Model file for the job. Use its own axes, mm. Round coordinates to 2 decimals unless told otherwise and drop trailing zeros. Loops run counter-clockwise (first coordinate to the right, second up) from the corner with the lowest first, then second, coordinate; pieces in that order, holes last. Notation, with made-up numbers: (3.25, -35.5) - (37.25, -35.5) arc R10 ccw to (37.25, -27.5) - close; hole circle Ø3 at (63, -38). An arc over 180 degrees is marked (long way). Answer as a JSON object with one key per item and string values.
from build123d import *

# Parameters (mm, degrees)
SKETCH1_W           = 396.875
SKETCH1_H           = 298.45
BOSS_EXTRUDE1_DEPTH = 2.38125
SKETCH5_R           = 1
CUT_EXTRUDE4_DEPTH  = 10
SKETCH6_R           = 2
SKETCH6_R_2         = 30
CUT_EXTRUDE5_DEPTH  = 10
SKETCH7_R           = 12.7
CUT_EXTRUDE6_DEPTH  = 10
CUT_EXTRUDE7_DEPTH  = 10


with BuildPart() as part:
    # Sketch1 → Boss-Extrude1 (new body)
    with BuildSketch(Plane(origin=(0, 0, 0), x_dir=(1, 0, 0), z_dir=(0, 1, 0))):
        Rectangle(SKETCH1_W, SKETCH1_H)
    extrude(amount=BOSS_EXTRUDE1_DEPTH)

    # Sketch5 → Cut-Extrude4 (cut)
    with BuildSketch(Plane.XZ):
        with Locations(Location((-138.4375, 138.55, 0), (0, 0, 270))):
            Circle(SKETCH5_R)
        with Locations(Location((-138.4375, -138.55, 0), (0, 0, 270))):
            Circle(SKETCH5_R)
        with Locations(Location((-131.4375, -121.05, 0), (0, 0, 270))):
            Circle(SKETCH5_R)
        with Locations(Location((-131.4375, 121.05, 0), (0, 0, 270))):
            Circle(SKETCH5_R)
        with Locations(Location((-145.4375, 121.05, 0), (0, 0, 270))):
            Circle(SKETCH5_R)
        with Locations(Location((-145.4375, -121.05, 0), (0, 0, 270))):
            Circle(SKETCH5_R)
    extrude(amount=-CUT_EXTRUDE4_DEPTH, mode=Mode.SUBTRACT)

    # Sketch6 → Cut-Extrude5 (cut)
    with BuildSketch(Plane(origin=(0, 2.38125, 0), x_dir=(1, 0, 0), z_dir=(0, 1, 0))):
        with Locations(Location((123.4375, 52.475, 0), (0, 0, 270))):
            Circle(SKETCH6_R)
        with Locations(Location((123.4375, -37.525, 0), (0, 0, 270))):
            Circle(SKETCH6_R)
        with Locations(Location((168.4375, 7.475, 0), (0, 0, 270))):
            Circle(SKETCH6_R)
        with Locations(Location((78.4375, 7.475, 0), (0, 0, 270))):
            Circle(SKETCH6_R)
        with Locations(Location((123.4375, 7.475, 0), (0, 0, 270))):
            Circle(SKETCH6_R_2)
    extrude(amount=-CUT_EXTRUDE5_DEPTH, mode=Mode.SUBTRACT)

    # Sketch7 → Cut-Extrude6 (cut)
    with BuildSketch(Plane(origin=(0, 2.38125, 0), x_dir=(1, 0, 0), z_dir=(0, 1, 0))):
        with Locations(Location((153.4375, 84.225, 0), (0, 0, 270))):
            Circle(SKETCH7_R)
    extrude(amount=-CUT_EXTRUDE6_DEPTH, mode=Mode.SUBTRACT)

    # Sketch8 → Cut-Extrude7 (cut)
    with BuildSketch(Plane(origin=(0, 2.38125, 0), x_dir=(1, 0, 0), z_dir=(0, 1, 0))):
        Polygon((131.7625, -149.225), (198.4375, -82.55), (198.4375, -149.225), align=None)
        Polygon((198.4375, 149.225), (131.7625, 149.225), (198.4375, 82.55), align=None)
    cut_extrude7 = extrude(amount=-CUT_EXTRUDE7_DEPTH, mode=Mode.SUBTRACT)

    # Mirror1: Cut-Extrude7 across plane
    add(cut_extrude7.mirror(Plane(origin=(0, 0, 0), x_dir=(0, 0, 1), z_dir=(1, 0, 0))), mode=Mode.SUBTRACT)


solid = part.part
1) Two-plate mould, pull along Z, no slides. Class faces 1 (the flat face through (-3, 2.381, -2)), 2 (the flat face through (164.633, 1.207, 116.354)), 3 (the cylindrical face through (94.15, 1.21, -13.98)): pulls with the +Z half, pulls with the -Z half, needs draft (parallel to the pull), parting line crosses it, or undercut.
Values follow:
{"face 1": "needs draft", "face 2": "pulls with the +Z half", "face 3": "undercut"}
2) Slice it at A-A on y = 1.85. Count the separate pieces of the cut face and the enclosed holes in it, then the cut area to 3 significant figures.
Values follow:
{"separate pieces": "1", "enclosed holes": "12", "area": "106,000 mm²"}
3) Drop flat-ended pins along their axis: P1, Ø1.6, axis at x = -138.44, z = -138.55, coming from the +Y side; P2, Ø6.5, axis at x = 78.44, z = -7.48, coming from the -Y side. Give the stop position or say it passes through.
Values follow:
{"P1": "through", "P2": "y = 0"}
4) Slice it at C-C on x = -157.5. List the corners of the cut face in (y, z).
Values follow:
{"outline": "(0, -123.49) - (2.38, -123.49) - (2.38, 123.49) - (0, 123.49) - close"}
5) Probe probe 1 along X at (y, z) = (1.1, 121.05); probe 2 along Z at (x, y) = (-141.5, 1); probe 3 along X at (y, z) = (1.8, -4.5). List the from-to ranges inside material, lowest first.
Values follow:
{"probe 1": "-159.94 to -146.44, -144.44 to -132.44, -130.44 to 159.94", "probe 2": "-139.49 to 139.49", "probe 3": "-198.44 to 93.59, 153.29 to 198.44"}
6) Slice it at B-B on z = -127. List the corners of the cut face in (x, y), then the cut area to 3 significant figures.
Values follow:
{"outline": "(-153.99, 0) - (153.99, 0) - (153.99, 2.38) - (-153.99, 2.38) - close", "area": "733 mm²"}
